Read the model definition and answer for the solid it produces. Units are mm, in the model's axes. A direction names the side the tool comes from. Give positions to 0.01 mm unless a question says otherwise; leave off trailing zeros. Order: outer loops, then holes, each group sorted by start corner. A loop starts at its lowest first (then second) coordinate and runs counter-clockwise, first axis right, second up.
Item 1: Given pin 1 Ø2 at (y, z) = (-6.5, 4) entering from +X; pin 2 Ø1 at (x, z) = (-3.5, -1.5) entering from +Y; pin 3 Ø3 at (y, z) = (-1.5, 3.5) entering from -X; pin 4 Ø2 at (y, z) = (-8.5, -0.5) entering from -X, each flat-ended and moving along its own axis, determine where each tip first touches the part or whether it passes through.
Item 2: Which of the six approach directions +Z, -Z, +X, -X, +Y, -Y give full straight-line access (tool end or side, diameter ignored) to faces 1 (the face through (-3.135, -2.404, 3.176)), 2 (the face through (0, 0, -2))?
Item 3: A cutting plane is placed at A-A (y = 0). Write down the section's boundary in (x, z).
Item 4: Find the intervals of material crossed by line 1 along Z through (x, y) = (0.5, 8.5); line 2 along Z through (x, y) = (-1.75, -4); line 3 along Y through (x, z) = (3.75, -1), in increasing order.
Item 5: A cutting plane is placed at D-D (z = -0.75). Write down the section's boundary in (x, y), plus the area to 3 significant figures.
Item 6: A cutting plane is placed at C-C (z = 2.5). Write down the section's boundary in (x, y), plus the area to 3 significant figures.
from build123d import *

# Parameters (mm, degrees)
F0_R     = 11
F0_R_2   = 5
F1_DEPTH = 2
F2_DEPTH = 1.5
F3_R     = 3.95
F4_DEPTH = 3.4


with BuildPart() as f1:
    # F0 (on Top) → F1 (new body)
    with BuildSketch(Plane.XY):
        Circle(F0_R)
        Circle(F0_R_2, mode=Mode.SUBTRACT)
        Circle(F0_R_2)
    extrude(amount=-F1_DEPTH)

    # F0 (on Top) → F2 (join)
    with BuildSketch(Plane.XY):
        Circle(F0_R_2)
    extrude(amount=F2_DEPTH)

    # F3 (on face) → F4 (join)
    with BuildSketch(Plane.XY.offset(1.5)):
        Circle(F3_R)
    extrude(amount=F4_DEPTH)


solid = f1.part
Response values:
1. pin 1: passes through
1. pin 2: stops at y = 10.58
1. pin 3: stops at x = -3.95
1. pin 4: stops at x = -8.05
2. face 1: +Z
2. face 2: -Z, +X, -X, +Y, -Y
3. outline: (-11, -2) - (11, -2) - (11, 0) - (5, 0) - (5, 1.5) - (3.95, 1.5) - (3.95, 4.9) - (-3.95, 4.9) - (-3.95, 1.5) - (-5, 1.5) - (-5, 0) - (-11, 0) - close
4. line 1: z = -2 to 0
4. line 2: z = -2 to 1.5
4. line 3: y = -10.34 to 10.34
5. outline: circle Ø22 at (0, 0)
5. area: 380 mm2
6. outline: circle Ø7.9 at (0, 0)
6. area: 49.0 mm2
